from build123d import *

# Parameters (mm, degrees)
F1_DEPTH = 9
F3_DEPTH = 9
F4_R     = 2.5
F5_DEPTH = 25


with BuildPart() as f1:
    # F0 (on Top) → F1 (new body)
    with BuildSketch(Plane.XY):
        Polygon((60, 145.017109), (-60, 145.017109), (-155.5885, -20.54703), (-95.5885, -124.470079), (95.5885, -124.470079), (155.5885, -20.54703), align=None)
    extrude(amount=F1_DEPTH)

    # F2 (on face) → F3 (join)
    with BuildSketch(Plane.XY.offset(9)):
        Polygon((-94.641016, 145.017109), (-172.909008, 9.45297), (-155.5885, -20.54703), (-60, 145.017109), align=None)
        Polygon((94.641016, 145.017109), (60, 145.017109), (155.5885, -20.54703), (172.909008, 9.45297), align=None)
        Polygon((95.5885, -124.470079), (-95.5885, -124.470079), (-78.267992, -154.470079), (78.267992, -154.470079), align=None)
    extrude(amount=-F3_DEPTH)

    # F4 (on face) → F5 (cut)
    with BuildSketch(Plane.XY.offset(9)):
        Circle(F4_R)
    extrude(amount=-F5_DEPTH, mode=Mode.SUBTRACT)


solid = f1.part
CAD build for the part. Positions are in the model's coordinates, mm. Round coordinates to 2 decimals unless told otherwise and drop trailing zeros. Write each loop counter-clockwise with the first axis right and the second up, starting at its lowest first coordinate (ties: lowest second). Pieces come first, ordered by that corner, then holes.
(1) Probe line 1 along Y through (x, z) = (0, 4.5); line 2 along Y through (x, z) = (-108, 8.25); line 3 along Y through (x, z) = (-94.5, 3). List the from-to ranges inside material, lowest first.
(2) Drop flat-ended pins along their axis: P1, Ø4.5, axis at x = 0, y = 0, coming from the -Z side; P2, Ø3, axis at y = -7.5, z = 2.5, coming from the +X side; P3, Ø2, axis at x = -92.5, z = 3.5, coming from the -Y side. Give the stop position or say it passes through.
(3) Slice it at A-A, the plane z = 5. Write the cut outline in (x, y), and give its area (3 significant figures).
(4) Slice it at B-B, the plane x = -125. Write the cut outline in (y, z), and give its area (3 significant figures).
(5) Slice it at C-C, the plane y = -67. Write the cut outline in (x, z).
From the geometry:
1. line 1: y = -154.47 to -2.5, 2.5 to 145.02
1. line 2: y = -102.97 to 121.88
1. line 3: y = -126.36 to 145.02
2. P1: passes through
2. P2: stops at x = 163.99
2. P3: stops at y = -131.55
3. outline: (-172.91, 9.45) - (-78.27, -154.47) - (78.27, -154.47) - (172.91, 9.45) - (94.64, 145.02) - (-94.64, 145.02) - close; hole circle Ø5 at (0, 0)
3. area: 77,400 mm2
4. outline: (-73.53, 0) - (92.43, 0) - (92.43, 9) - (-73.53, 9) - close
4. area: 1,490 mm2
5. outline: (-128.77, 0) - (128.77, 0) - (128.77, 9) - (-128.77, 9) - close
